Geometry: final body of the model. Coordinates: model frame, mm. Coordinates: 2 decimals unless noted, no trailing zeros. Write each loop counter-clockwise with the first axis right and the second up, starting at its lowest first coordinate (ties: lowest second). Pieces come first, ordered by that corner, then holes. Notation, with made-up numbers: (22, -10) - (64, -10) arc R17 ccw to (64, 10) - close; hole circle Ø8 at (46, 14). An arc over 180 degrees is marked (long way). Answer as a JSON object with one key per item and string values. Group by question number.
Item 1: Section B-B on y = 32. Return loops of the section in (x, z).
Item 2: Section D-D on y = 21. Return loops of the section in (x, z), and give its area (3 significant figures).
Item 3: Section C-C on x = -13.5. Return loops of the section in (y, z), and give its area (3 significant figures).
Item 4: Section A-A on x = 2.5. Return loops of the section in (y, z), and give its area (3 significant figures).
Item 5: First-contact query: pin 1 Ø1.8 at (x, y) = (-5.24, 58) entering from +Z; pin 2 Ø1.5 at (y, z) = (6.5, 0.5) entering from -X. Flat tips, straight axial feed; report the tip coordinate or a pass-through.
Item 6: Line query: line 1 along X through (y, z) = (17, 1.7); line 2 along Y through (x, z) = (-6, 1.05); line 3 along Y through (x, z) = (4, 0.95). Output: solid intervals per line, ascending. Write a range as from..to.
```python
from build123d import *

# Parameters (mm, degrees)
SKETCH_1_R      = 8.5
SKETCH_1_R_2    = 1.5
SKETCH_1_W      = 17.460607986
SKETCH_1_H      = 3
EXTRUDE_1_DEPTH = 3


with BuildPart() as part:
    # 스케치1 → 보스-돌출1 (new body)
    # profile 1 of 2: a face of its own
    with BuildSketch(Plane.XY):
        Polygon((20.5, 17.599715907), (20.5, 47.899715907), (7.989824602, 62), (-7.989824602, 62), (-20.5, 47.899715907), (-20.5, 17.599715907), (-11, 0), (11, 0), align=None)
        with Locations((7.5, 17.599715907)):
            Circle(SKETCH_1_R, mode=Mode.SUBTRACT)
        with Locations((13.5, 37.599715907)):
            Circle(SKETCH_1_R_2, mode=Mode.SUBTRACT)
        with Locations((-5.239824602, 58)):
            Circle(SKETCH_1_R_2, mode=Mode.SUBTRACT)
        with Locations((-6, 4)):
            Circle(SKETCH_1_R_2, mode=Mode.SUBTRACT)
        with Locations((-13.5, 37.599715907)):
            Circle(SKETCH_1_R_2, mode=Mode.SUBTRACT)
        with Locations((6, 4)):
            Circle(SKETCH_1_R_2, mode=Mode.SUBTRACT)
        with Locations((5.239824602, 58)):
            Circle(SKETCH_1_R_2, mode=Mode.SUBTRACT)
        with BuildLine():
            ThreePointArc((11.156743405, 29.02898656), (13.621468977, 30.35740093), (12.202349665, 32.771040767))
            ThreePointArc((12.202349665, 32.771040767), (10.039769884, 33.990449008), (8.730303993, 36.099715907))
            Line((8.730303993, 36.099715907), (8.730303993, 39.099715907))
            ThreePointArc((8.730303993, 39.099715907), (10.039769884, 41.208982805), (12.202349665, 42.428391047))
            ThreePointArc((12.202349665, 42.428391047), (0, 50.15321463), (-12.202349665, 42.428391047))
            ThreePointArc((-12.202349665, 42.428391047), (-10.039769884, 41.208982805), (-8.730303993, 39.099715907))
            Line((-8.730303993, 39.099715907), (-8.730303993, 36.099715907))
            ThreePointArc((-8.730303993, 36.099715907), (-10.181651088, 33.8595875), (-12.578672362, 32.685333404))
            Line((-12.578672362, 32.685333404), (-12.578672362, 19.505123412))
            ThreePointArc((-12.578672362, 19.505123412), (-8.463216291, 15.389667341), (-4.34776022, 19.505123412))
            ThreePointArc((-4.34776022, 19.505123412), (1.219141664, 27.824725372), (11.156743405, 29.02898656))
        make_face(mode=Mode.SUBTRACT)
    # profile 2 of 2: a face of its own
    with BuildSketch(Plane.XY):
        with Locations((0, 37.599715907)):
            Rectangle(SKETCH_1_W, SKETCH_1_H)
    extrude(amount=EXTRUDE_1_DEPTH)


solid = part.part
```
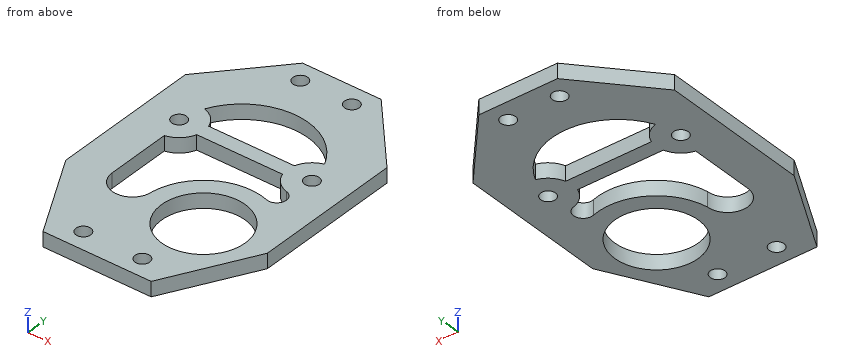
Checks:
{
 "1": {"outline": "(-20.5, 0) - (-12.58, 0) - (-12.58, 3) - (-20.5, 3) - close; (13.34, 0) - (20.5, 0) - (20.5, 3) - (13.34, 3) - close"},
 "2": {"outline": "(-20.5, 0) - (-12.58, 0) - (-12.58, 3) - (-20.5, 3) - close; (-4.01, 0) - (-0.29, 0) - (-0.29, 3) - (-4.01, 3) - close; (15.29, 0) - (20.5, 0) - (20.5, 3) - (15.29, 3) - close", "area": "50.5 mm^2"},
 "3": {"outline": "(4.63, 0) - (36.1, 0) - (36.1, 3) - (4.63, 3) - close; (39.1, 0) - (55.79, 0) - (55.79, 3) - (39.1, 3) - close", "area": "144 mm^2"},
 "4": {"outline": "(0, 0) - (10.73, 0) - (10.73, 3) - (0, 3) - close; (24.47, 0) - (28.51, 0) - (28.51, 3) - (24.47, 3) - close; (36.1, 0) - (39.1, 0) - (39.1, 3) - (36.1, 3) - close; (49.92, 0) - (62, 0) - (62, 3) - (49.92, 3) - close", "area": "89.5 mm^2"},
 "5": {"pin 1": "through", "pin 2": "x = -14.91"},
 "6": {"line 1": "-20.18..-11.73, -5.2..-0.98, 15.98..20.18", "line 2": "0..2.5, 5.5..16.21, 36.1..39.1, 48.75..56.71, 59.29..62", "line 3": "0..9.85, 25.35..29.08, 36.1..39.1, 49.55..57.16, 58.84..62"}
}
